Check sheet for the modelled part. Datum: model origin and axes. Units: mm. Face numbers are marked on the shaded views. A direction names the side the tool comes from. Round coordinates to 2 decimals unless told otherwise and drop trailing zeros. Order: outer loops, then holes, each group sorted by start corner. A loop starts at its lowest first (then second) coordinate and runs counter-clockwise, first axis right, second up.
Q1. Cross-section at A-A on x = 86. Record the cut outline in (y, z).
Q2. Cross-section at D-D on x = 46. Record the cut outline in (y, z), then the cut area to 3 significant figures.
Q3. Scan lines: probe 1 along Y at (x, z) = (36.2, 26.2); probe 2 along X at (y, z) = (118.95, 26.05); probe 3 along Z at (x, y) = (15.5, 110.25). Record each from-to range of solid material in increasing order.
Q4. Mould release check, pull along Z, two halves, no side actions. Record for the marked faces 3, 4, 5 and 6: +Z half, -Z half, draft (parallel to the pull), parting line (faces both ways), or undercut.
Q5. Set-up check for the marked faces 1 and 2: record each of +Z, -Z, +X, -X, +Y, -Y from which the full face is reachable in a straight line by a thin tool's end or side.
Q6. Cross-section at B-B on z = 14. Give the number of separate pieces and of enclosed holes in the cut face, then the cut area to 3 significant figures.
Q7. Cross-section at C-C on y = 106. Record the cut outline in (x, z).
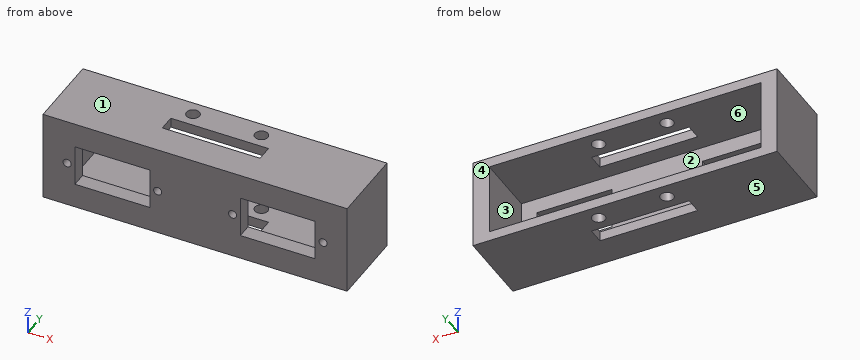
Autodesk Inventor part; units mm, degrees
ref_plane "YZ Plane" through (0, 0, 0) normal (1, 0, 0) x (0, 1, 0)
ref_plane "XZ Plane" through (0, 0, 0) normal (0, 1, 0) x (-1, 0, 0)
ref_plane "XY Plane" through (0, 0, 0) normal (0, 0, 1) x (1, 0, 0)
sketch "Sketch1" plane through (0, 0, 0) normal (0, 0, 1) x (1, 0, 0)
  line L0 (0, 0) -> (93.4, 0)
  line L1 (93.4, 0) -> (93.4, 100)
  line L2 (93.4, 100) -> (0, 100)
  line L3 (0, 100) -> (0, 0)
  dimension "d0" = 93.4
  dimension "d1" = 100
extrude "Extrusion1" add sketch "Sketch1" along normal blind 3
sketch "Sketch2" plane through (0, 100, 0) normal (0, 1, 0) x (1, 0, 0)
  line L0 (0, 0) -> (0, -3)
  line L1 (0, 0) -> (93.4, 0)
  line L2 (93.4, 0) -> (93.4, -28)
  line L3 (93.4, -28) -> (0, -28)
  line L4 (0, -28) -> (0, 0)
  line L5 (93.4, 0) -> (0, 0)
  line L6 (0, 0) -> (0, -3)
  line L7 (93.4, -3) -> (0, -3)
  line L8 (93.4, 0) -> (93.4, -3)
  line L9 (93.4, -3) -> (0, -3)
  line L10 (83.6, -20.35) -> (60.6, -20.35)
  line L11 (60.6, -20.35) -> (60.6, -7.65)
  line L12 (60.6, -7.65) -> (83.6, -7.65)
  line L13 (83.6, -7.65) -> (83.6, -20.35)
  line L14 (32.8, -7.65) -> (9.8, -7.65)
  line L15 (9.8, -7.65) -> (9.8, -20.35)
  line L16 (9.8, -20.35) -> (32.8, -20.35)
  line L17 (32.8, -20.35) -> (32.8, -7.65)
  arc A0 (86.9526, -8.8) -> (86.9526, -9.9) centre (86, -9.35) ccw
  arc A1 (57.2474, -9.9) -> (57.2474, -8.8) centre (58.2, -9.35) ccw
  arc A2 (36.1526, -8.8) -> (36.1526, -9.9) centre (35.2, -9.35) ccw
  arc A3 (6.4474, -9.9) -> (6.4474, -8.8) centre (7.4, -9.35) ccw
  circle A4 centre (7.4, -14) radius 1.25
  circle A5 centre (35.2, -14) radius 1.25
  circle A6 centre (58.2, -14) radius 1.25
  circle A7 centre (86, -14) radius 1.25
  point P0 (9.8, -3)
  point P1 (32.8, -3)
  point P2 (60.6, -3)
  point P3 (83.6, -3)
  point P4 (32.8, -14)
  dimension "d4" = 3
  dimension "d6" = 9.8
  dimension "d7" = 7.65
  dimension "d8" = 23
  dimension "d9" = 9.8
  dimension "d13" = 12.7
  dimension "d14" = 28
  dimension "d15" = 7.65
  dimension "d16" = 2.5
extrude "Extrusion2" add sketch "Sketch2" along normal blind 4.5
sketch "Sketch3" plane through (0, 104.5, 0) normal (0, 1, 0) x (1, 0, 0)
  line L0 (93.4, -28) -> (93.4, 0)
  line L1 (93.4, 0) -> (0, 0)
  line L2 (0, 0) -> (0, -28)
  line L3 (0, -28) -> (93.4, -28)
  circle A0 centre (86, -14) radius 1.25
  circle A1 centre (7.4, -14) radius 1.25
  circle A2 centre (35.2, -14) radius 1.25
  circle A3 centre (58.2, -14) radius 1.25
  line L4 (32.8, -7.65) -> (32.8, -20.35)
  line L5 (32.8, -20.35) -> (9.8, -20.35)
  line L6 (9.8, -20.35) -> (9.8, -7.65)
  line L7 (9.8, -7.65) -> (32.8, -7.65)
  line L8 (83.6, -20.35) -> (60.6, -20.35)
  line L9 (60.6, -20.35) -> (60.6, -7.65)
  line L10 (60.6, -7.65) -> (83.6, -7.65)
  line L11 (83.6, -7.65) -> (83.6, -20.35)
  line L12 (88.4, -25) -> (5, -25)
  line L13 (5, -25) -> (5, -3)
  line L14 (5, -3) -> (88.4, -3)
  line L15 (88.4, -3) -> (88.4, -25)
  point P0 (88.4, -14)
  point P1 (93.4, -14)
  dimension "d17" = 5
  dimension "d18" = 5
  dimension "d19" = 22
extrude "Extrusion3" add sketch "Sketch3" along normal blind 19 contours L3 L2 L1 L0
sketch "Sketch4" plane through (0, 100, 28) normal (0, 0, 1) x (1, 0, 0)
  line L0 (0, 0) -> (93.4, 0)
  line L1 (93.4, 0) -> (93.4, 23.5)
  line L2 (0, 23.5) -> (93.4, 23.5)
  line L3 (0, 0) -> (0, 23.5)
  point P0 (0, -100)
  point P1 (36.2, 18.95)
  point P2 (46.7, 23.5)
  point P3 (57.2, 18.95)
  dimension "d23" = 36.2
  dimension "d24" = 36.2
  dimension "d25" = 4.55
hole "Hole1" at (36.2, 118.95, 28) at (57.2, 118.95, 28) direction (0, 0, -1) diameter 4 end through all
sketch "Sketch5" plane through (0, 100, 28) normal (0, 0, 1) x (1, 0, 0)
  circle A0 centre (36.2, 18.95) radius 2
  circle A1 centre (57.2, 18.95) radius 2
  line L0 (0, 0) -> (93.4, 0)
  line L1 (93.4, 0) -> (93.4, 23.5)
  line L2 (0, 23.5) -> (93.4, 23.5)
  line L3 (0, 0) -> (0, 23.5)
  line L4 (61.7, 9.5) -> (31.7, 9.5)
  line L5 (31.7, 9.5) -> (31.7, 14.5)
  line L6 (31.7, 14.5) -> (61.7, 14.5)
  line L7 (61.7, 14.5) -> (61.7, 9.5)
  point P0 (0, -100)
  point P1 (46.7, 14.5)
  point P2 (46.7, 23.5)
  dimension "d33" = 9
  dimension "d34" = 14
  dimension "d35" = 30
extrude "Extrusion4" cut sketch "Sketch5" against normal through all contours L4 L5 L6 L7
sketch "Sketch6" plane through (0, 0, 3) normal (0, 0, 1) x (1, 0, 0)
  line L0 (93.4, 0) -> (93.4, 100)
  line L1 (93.4, 100) -> (0, 100)
  line L2 (0, 100) -> (0, 0)
  line L3 (0, 0) -> (93.4, 0)
extrude "Extrusion5" cut sketch "Sketch6" against normal blind 10
equation "\"d7\" = d15"
equation "\"d9\" = d6"
equation "\"d18\" = d17"
properties part number "Frame"
Results found:
1. outline: (100, 0) - (123.5, 0) - (123.5, 3) - (104.5, 3) - (104.5, 12.75) - (100, 12.75) - close; (100, 15.25) - (104.5, 15.25) - (104.5, 25) - (123.5, 25) - (123.5, 28) - (100, 28) - close
2. outline: (100, 0) - (109.5, 0) - (109.5, 3) - (104.5, 3) - (104.5, 25) - (109.5, 25) - (109.5, 28) - (100, 28) - close; (114.5, 0) - (123.5, 0) - (123.5, 3) - (114.5, 3) - close; (114.5, 25) - (123.5, 25) - (123.5, 28) - (114.5, 28) - close
2. area: 210 mm2
3. probe 1: y = 100 to 109.5, 114.5 to 116.95, 120.95 to 123.5
3. probe 2: x = 0 to 34.2, 38.2 to 55.2, 59.2 to 93.4
3. probe 3: z = 0 to 3, 25 to 28
4. face 3: undercut
4. face 4: draft
4. face 5: -Z half
4. face 6: undercut
5. face 1: +Z, +X, -X, +Y, -Y
5. face 2: +Y
6. separate pieces: 7
6. enclosed holes: 0
6. area: 358 mm2
7. outline: (0, 0) - (93.4, 0) - (93.4, 28) - (0, 28) - close; hole (5, 3) - (88.4, 3) - (88.4, 25) - (5, 25) - close
